Autodesk Fusion 360 part; units mm, degrees
sketch "Sketch1" plane through (0, 0, 0) normal (0, 0, 1) x (1, 0, 0)
  line L0 (0, 0) -> (40, 0)
  line L1 (40, 0) -> (40, 40)
  line L2 (40, 40) -> (0, 40)
  line L3 (0, 40) -> (0, 0)
  dimension "d1" = 40
  dimension "d2" = 40
sketch "Sketch2" plane through (0, 0, 0) normal (0, 0, 1) x (1, 0, 0)
  circle A0 centre (10, 31) radius 3
  circle A1 centre (30, 31) radius 3
  circle A2 centre (10, 10) radius 3
  circle A3 centre (30, 11) radius 3
  line L0 (0, 40) -> (0, 0)
  line L1 (40, 0) -> (40, 40)
  line L2 (40, 40) -> (0, 40)
  line L3 (0, 0) -> (40, 0)
  dimension "d3" = 6
  dimension "d4" = 6
  dimension "d5" = 6
  dimension "d6" = 6
  dimension "d7" = 10
  dimension "d8" = 10
  dimension "d9" = 10
  dimension "d10" = 10
  dimension "d11" = 9
  dimension "d12" = 9
  dimension "d13" = 10
  dimension "d14" = 11
extrude "Extrude1" add sketch "Sketch2" along normal blind 3
sketch "Sketch3" plane through (0, 0, 3) normal (0, 0, 1) x (-1, 0, 0)
  circle A0 centre (-30, -31) radius 3
  circle A1 centre (-30, -11) radius 3
  circle A2 centre (-10, -31) radius 3
  circle A3 centre (-10, -10) radius 3
  line L0 (0, 0) -> (-40, 0)
  line L1 (-40, 0) -> (-40, -40)
  line L2 (-40, -40) -> (0, -40)
  line L3 (0, -40) -> (0, 0)
  circle A4 centre (-10, -31) radius 4.3
  circle A5 centre (-30, -31) radius 4.3
  circle A6 centre (-10, -10) radius 4.3
  circle A7 centre (-30, -11) radius 4.3
  line L4 (0, -40) -> (-40, -40)
  line L5 (-40, -40) -> (-40, 0)
  line L6 (-40, 0) -> (0, 0)
  line L7 (0, 0) -> (0, -40)
  dimension "d17" = 8.6
  dimension "d18" = 8.6
  dimension "d19" = 8.6
  dimension "d20" = 8.6
extrude "Extrude2" add sketch "Sketch3" along normal blind 5 contours L0 L1 L2 L3 L4 L5 L6 L7
sketch "Sketch4" plane through (0, 0, 8) normal (0, 0, 1) x (-1, 0, 0)
  circle A0 centre (-30, -11) radius 4.3
  circle A1 centre (-30, -31) radius 4.3
  circle A2 centre (-10, -31) radius 4.3
  circle A3 centre (-10, -10) radius 4.3
  line L0 (0, 0) -> (-40, 0)
  line L1 (-40, 0) -> (-40, -40)
  line L2 (-40, -40) -> (0, -40)
  line L3 (0, -40) -> (0, 0)
  line L4 (-40, -40) -> (-37, -40)
  line L5 (-37, -40) -> (-37, 0)
  line L6 (-37, 0) -> (-40, 0)
  line L7 (-40, 0) -> (-40, -40)
  line L8 (0, -40) -> (-3, -40)
  line L9 (-3, -40) -> (-3, 0)
  line L10 (-3, 0) -> (0, 0)
  line L11 (0, 0) -> (0, -40)
  line L12 (0, -40) -> (-40, -40)
  line L13 (-40, -40) -> (-40, -37)
  line L14 (-40, -37) -> (0, -37)
  line L15 (0, -37) -> (0, -40)
  line L16 (0, 0) -> (-40, 0)
  line L17 (-40, 0) -> (-40, -3)
  line L18 (-40, -3) -> (0, -3)
  line L19 (0, -3) -> (0, 0)
  dimension "d23" = 3
  dimension "d24" = 40
  dimension "d25" = 3
  dimension "d26" = 3
  dimension "d27" = 3
extrude "Extrude3" add sketch "Sketch4" along normal blind 100 contours L0 L3 L9 L10 L11 L16 L18 L19 | L0 L5 L9 L16 L18 | L3 L9 L11 L14 L18 | L0 L1 L5 L6 L7 L16 L17 L18 | L2 L3 L8 L9 L11 L12 L14 L15 | L1 L5 L7 L14 L18 | L2 L5 L9 L12 L14 | L1 L2 L4 L5 L7 L12 L13 L14
sketch "Sketch5" plane through (0, 0, 0) normal (0, -1, 0) x (1, 0, 0)
  line L0 (0, 0) -> (40, 0)
  line L1 (40, 0) -> (40, 108)
  line L2 (40, 108) -> (0, 108)
  line L3 (0, 108) -> (0, 0)
sketch "Sketch6" plane through (0, 0, 0) normal (-1, 0, 0) x (0, -1, 0)
  line L0 (-40, 0) -> (0, 0)
  line L1 (0, 0) -> (0, 108)
  line L2 (0, 108) -> (-40, 108)
  line L3 (-40, 108) -> (-40, 0)
  line L4 (-3, 8) -> (-37, 8)
  line L5 (-37, 8) -> (-37, 98)
  line L6 (-37, 98) -> (-3, 98)
  line L7 (-3, 98) -> (-3, 8)
  line L8 (-40, 0) -> (0, 0)
  dimension "d30" = 3
  dimension "d31" = 3
  dimension "d32" = 8
  dimension "d33" = 90
extrude "Extrude4" cut sketch "Sketch6" against normal blind 10 contours L4 L5 L6 L7
sketch "Sketch7" plane through (0, 0, 108) normal (0, 0, 1) x (-1, 0, 0)
  line L0 (-3, -3) -> (-3, -37)
  line L1 (-3, -37) -> (-37, -37)
  line L2 (-37, -37) -> (-37, -3)
  line L3 (-37, -3) -> (-3, -3)
  line L4 (0, -40) -> (0, 0)
  line L5 (0, 0) -> (-40, 0)
  line L6 (-40, 0) -> (-40, -40)
  line L7 (-40, -40) -> (0, -40)
  line L8 (-3, -37) -> (-37, -37)
  line L9 (-37, -37) -> (-37, -3)
  line L10 (-37, -3) -> (-3, -3)
  line L11 (-3, -3) -> (-3, -37)
extrude "Extrude5" add sketch "Sketch7" against normal blind 3 contours L0 L1 L2 L3 L8 L9 L10 L11
sketch "Sketch8" plane through (0, 0, 0) normal (0, -1, 0) x (1, 0, 0)
  line L0 (9, 88) -> (31, 88)
  line L1 (31, 88) -> (31, 70)
  line L2 (31, 70) -> (9, 70)
  line L3 (9, 70) -> (9, 88)
  line L4 (0, 108) -> (0, 0)
  line L5 (40, 0) -> (40, 108)
  line L6 (40, 108) -> (0, 108)
  line L7 (0, 0) -> (40, 0)
  dimension "d38" = 9
  dimension "d39" = 9
  dimension "d40" = 20
  dimension "d41" = 70
extrude "Extrude6" cut sketch "Sketch8" against normal blind 15 contours L0 L1 L2 L3
sketch "Sketch9" plane through (0, 0, 0) normal (-1, 0, 0) x (0, -1, 0)
  line L0 (-37, 8) -> (-37, 98)
  line L1 (-37, 98) -> (-3, 98)
  line L2 (-3, 98) -> (-3, 8)
  line L3 (-3, 8) -> (-37, 8)
  line L4 (-40, 0) -> (0, 0)
  line L5 (0, 0) -> (0, 108)
  line L6 (0, 108) -> (-40, 108)
  line L7 (-40, 108) -> (-40, 0)
Design review of the part built by this model. Coordinates are the model's own, in mm. A direction names the side the tool comes from. Round coordinates to 2 decimals unless told otherwise and drop trailing zeros. Write each loop counter-clockwise with the first axis right and the second up, starting at its lowest first coordinate (ties: lowest second). Pieces come first, ordered by that corner, then holes. Notation, with made-up numbers: (62.5, 52.5) - (105.5, 52.5) arc R9 ccw to (105.5, 60.5) - close; hole circle Ø7 at (48, 58). An arc over 180 degrees is marked (long way). Use a Markdown table: item, result. Add a question column.
1. Wall thickness on probe 1 along Y at (x, z) = (30, 5.7); probe 2 along Y at (x, z) = (30, 2.45); probe 3 along X at (y, z) = (31, 5.65): over which ranges is each line inside the solid? List them lowest first.
2. For faces 5 (the face through (27, 10, 3)), 6 (the face through (20, 1, 88)), 7 (the face through (12.86, 30.1, 1.48)), 8 (the face through (1, 20, 98)), list the 3-axis set-ups (+Z, -Z, +X, -X, +Y, -Y) from which the entire face can be reached by the end or side of a thin tool; tool diameter is ignored.
3. We need section C-C (z = 84.5). State the section outline as (x, y) points.
4. Mouldability with a two-part tool opening along X and no side actions: class faces 1 (the face through (25.9, 12.3, 5.5)), 2 (the face through (18, 20, 8)), 3 (the face through (40, 20, 53)), 4 (the face through (28.016, 27.185, 5.465)) as +X half, -X half, draft (parallel to the pull), parting line (faces both ways), or undercut.
5. Clearance check with a flat-ended pin moving along its axis: pin 1 (3.5 mm diameter, centred on x = 10, y = 10, fed in from -Z). State where the tip first meets the part, or that it passes through.
6. We need section D-D (z = 56). State the section outline as (x, y) points, then the cut area to 3 significant figures.
7. We need section B-B (y = 31). State the section outline as (x, z) points, then the cut area to 3 significant figures.
8. We need section A-A (x = 30). State the section outline as (y, z) points, then the cut area to 3 significant figures.
Output:
| question | item | result |
|---|---|---|
| 1 | probe 1 | y = 0 to 6.7, 15.3 to 26.7, 35.3 to 40 |
| 1 | probe 2 | y = 0 to 8, 14 to 28, 34 to 40 |
| 1 | probe 3 | x = 0 to 5.7, 14.3 to 25.7, 34.3 to 40 |
| 2 | face 5 | none |
| 2 | face 6 | -Y |
| 2 | face 7 | -Z |
| 2 | face 8 | -X |
| 3 | outline | (0, 0) - (9, 0) - (9, 3) - (0, 3) - close; (0, 37) - (37, 37) - (37, 3) - (31, 3) - (31, 0) - (40, 0) - (40, 40) - (0, 40) - close |
| 4 | face 1 | undercut |
| 4 | face 2 | draft |
| 4 | face 3 | +X half |
| 4 | face 4 | undercut |
| 5 | pin 1 | stops at z = 105 |
| 6 | outline | (0, 0) - (40, 0) - (40, 40) - (0, 40) - (0, 37) - (37, 37) - (37, 3) - (0, 3) - close |
| 6 | area | 342 mm2 |
| 7 | outline | (0, 0) - (7, 0) - (7, 3) - (5.7, 3) - (5.7, 8) - (0, 8) - close; (0, 98) - (3, 98) - (3, 105) - (37, 105) - (37, 8) - (34.3, 8) - (34.3, 3) - (33, 3) - (33, 0) - (40, 0) - (40, 108) - (0, 108) - close; (13, 0) - (27, 0) - (27, 3) - (25.7, 3) - (25.7, 8) - (14.3, 8) - (14.3, 3) - (13, 3) - close |
| 7 | area | 630 mm2 |
| 8 | outline | (0, 0) - (8, 0) - (8, 3) - (6.7, 3) - (6.7, 8) - (3, 8) - (3, 70) - (0, 70) - close; (0, 88) - (3, 88) - (3, 105) - (37, 105) - (37, 8) - (35.3, 8) - (35.3, 3) - (34, 3) - (34, 0) - (40, 0) - (40, 108) - (0, 108) - close; (14, 0) - (28, 0) - (28, 3) - (26.7, 3) - (26.7, 8) - (15.3, 8) - (15.3, 3) - (14, 3) - close |
| 8 | area | 846 mm2 |
